Build history of the part. All positions in model axes, mm. A direction names the side the tool comes from. Coordinates: 2 decimals unless noted, no trailing zeros. Write each loop counter-clockwise with the first axis right and the second up, starting at its lowest first coordinate (ties: lowest second). Pieces come first, ordered by that corner, then holes. Notation, with made-up numbers: (18.25, 78) -> (72.25, 78) arc R11 cw to (72.25, 98) -> close; hole circle Ø5 at (0, 82). An arc over 180 degrees is marked (long way). Write each question's results on one line, items separated by ' | '. Start each with the question number.
Q1. Drill centre lines: line 1 (Z direction, x = -4.75, y = 4.75); line 2 (Y direction, x = 2, z = 0); line 3 (Y direction, x = 0.75, z = 0). Where is each one in solid material? Low to high.
Q2. Saw through at A-A on x = 5.5. Give the cut face in (y, z), and give its area (3 significant figures).
Q3. Tool access for faces 1 (the face through (-3.9, 4.7, 1)), 2 (the face through (4, 3, -2.25)), 3 (the face through (0, 0, 0)): list every direction of +Z, -Z, +X, -X, +Y, -Y with a clear straight run to the whole face (end or side of a thin tool).
Q4. Saw through at C-C on x = -3.25. Give the cut face in (y, z).
Q5. Saw through at B-B on y = -0.25. Give the cut face in (x, z).
Q6. Drop a flat-ended pin along its axis: pin 1 Ø1.2 at (x, y) = (-2.5, 2.5) entering from -Z. Give the stop position or say it passes through.
Q7. Two-plate mould, pull along Z, no slides. Class faces 4 (the face through (-4.85, 0.6, 2.5)), 5 (the face through (7.2, 1, -1.5)), 6 (the face through (5, 3, -3.25)), 7 (the face through (-4, 3.8, 2.5)): released by +Z, released by -Z, zero draft, split by the parting line, or undercut.
from build123d import *
from build123d.topology import SkipClean

# Parameters (mm, degrees)
SKETCH1_W                            = 11.7
SKETCH1_H                            = 6.5
BOSS_EXTRUDE1_DEPTH                  = 5.5
SKETCH2_R                            = 1.75
CUT_EXTRUDE1_DEPTH                   = 15.5
BOSS_EXTRUDE2_START                  = 2.6
SKETCH3_R                            = 2.5
SKETCH3_R_2                          = 1.75
BOSS_EXTRUDE2_DEPTH                  = 2.6
CUT_EXTRUDE2_START                   = -1
CUT_EXTRUDE2_DEPTH                   = 9.7
CUT_EXTRUDE3_DEPTH                   = 10
SKETCH6_W                            = 2.5
SKETCH6_H                            = 2
SKETCH6_W_2                          = 2
CUT_EXTRUDE4_DEPTH                   = 2
SKETCH7_W                            = 9.85
SKETCH7_H                            = 4.5
CUT_EXTRUDE5_DEPTH                   = 0.5
FILLET1_R                            = 0.2
SKETCH8_R                            = 0.5
BOSS_EXTRUDE3_DEPTH                  = 1
BOSS_EXTRUDE3_DIRECTION_2_REACH      = 12.593
BOSS_EXTRUDE3_DIRECTION_2_END_RADIUS = 3
FILLET2_R                            = 0.3


with BuildPart() as part:
    # Sketch1 → Boss-Extrude1 (new body)
    with BuildSketch(Plane(origin=(0, 0, 0), x_dir=(1, 0, 0), z_dir=(0, 1, 0))):
        Rectangle(SKETCH1_W, SKETCH1_H)
    extrude(amount=BOSS_EXTRUDE1_DEPTH)

    # Sketch2 → Cut-Extrude1 (cut)
    with BuildSketch(Plane(origin=(5.85, 0, 0), x_dir=(0, 0, -1), z_dir=(1, 0, 0))):
        with Locations((0, 3)):
            Circle(SKETCH2_R)
    extrude(amount=-CUT_EXTRUDE1_DEPTH, mode=Mode.SUBTRACT)

    # Sketch3 → Boss-Extrude2 (add)
    with BuildSketch(Plane(origin=(5.85, 0, 0), x_dir=(0, 0, -1), z_dir=(1, 0, 0)).offset(BOSS_EXTRUDE2_START)):
        with Locations(Location((0, 3, 0), (0, 0, 90))):
            Circle(SKETCH3_R)
        with Locations((0, 3)):
            Circle(SKETCH3_R_2, mode=Mode.SUBTRACT)
    extrude(amount=-BOSS_EXTRUDE2_DEPTH)

    # Sketch4 → Cut-Extrude2 (cut)
    with BuildSketch(Plane(origin=(5.85, 0, 0), x_dir=(0, 0, -1), z_dir=(1, 0, 0)).offset(CUT_EXTRUDE2_START)):
        with BuildLine():
            Line((-4.687033743, 2), (-2.828427125, 2))
            ThreePointArc((-2.828427125, 2), (0, 0), (2.828427125, 2))
            Line((2.828427125, 2), (5.329187563, 2))
            Line((5.329187563, 2), (5.329187563, -1.490759496))
            Line((5.329187563, -1.490759496), (-4.687033743, -1.490759496))
            Line((-4.687033743, -1.490759496), (-4.687033743, 2))
        make_face()
    extrude(amount=-CUT_EXTRUDE2_DEPTH, mode=Mode.SUBTRACT)

    # Sketch5 → Cut-Extrude3 (cut)
    with BuildSketch(Plane(origin=(0, 5.5, 0), x_dir=(1, 0, 0), z_dir=(0, 1, 0))):
        Polygon((-3.5, 4.45), (-2, 4.45), (-2, 2.75), (-1.5, 2.75), (-1.5, 2.25), (-4, 2.25), (-4, 2.75), (-3.5, 2.75), align=None)
        Polygon((0.3, 4.45), (1.3, 4.45), (1.3, 2.75), (1.8, 2.75), (1.8, 2.25), (-0.2, 2.25), (-0.2, 2.75), (0.3, 2.75), align=None)
        Polygon((3.6, 4.45), (4.6, 4.45), (4.6, 2.75), (5.1, 2.75), (5.1, 2.25), (3.1, 2.25), (3.1, 2.75), (3.6, 2.75), align=None)
        Polygon((1.3, -2.75), (1.8, -2.75), (1.8, -2.25), (-0.2, -2.25), (-0.2, -2.75), (0.3, -2.75), (0.3, -4.45), (1.3, -4.45), align=None)
        Polygon((-2, -2.75), (-1.5, -2.75), (-1.5, -2.25), (-4, -2.25), (-4, -2.75), (-3.5, -2.75), (-3.5, -4.45), (-2, -4.45), align=None)
        Polygon((5.1, -2.25), (5.1, -2.75), (4.6, -2.75), (4.6, -4.45), (3.6, -4.45), (3.6, -2.75), (3.1, -2.75), (3.1, -2.25), align=None)
    extrude(amount=-CUT_EXTRUDE3_DEPTH, mode=Mode.SUBTRACT)

    # Sketch6 → Cut-Extrude4 (cut)
    with BuildSketch(Plane(origin=(0, 5.5, 0), x_dir=(1, 0, 0), z_dir=(0, 1, 0))):
        with Locations((-3.63, 0)):
            Rectangle(SKETCH6_W, SKETCH6_H)
        with Locations((0.9, 0)):
            Rectangle(SKETCH6_W_2, SKETCH6_H)
        with Locations((4.02, 0)):
            Rectangle(SKETCH6_W_2, SKETCH6_H)
    extrude(amount=-CUT_EXTRUDE4_DEPTH, mode=Mode.SUBTRACT)

    # Sketch7 → Cut-Extrude5 (cut)
    with BuildSketch(Plane(origin=(0, 5.5, 0), x_dir=(1, 0, 0), z_dir=(0, 1, 0))):
        with Locations((0.925, 0)):
            Rectangle(SKETCH7_W, SKETCH7_H)
    extrude(amount=-CUT_EXTRUDE5_DEPTH, mode=Mode.SUBTRACT)

    # Fillet1
    fillet1_edges = [part.edges().sort_by_distance(p)[0] for p in [
        (-2.75, 5, -2.25),
        (0.8, 5, -2.25),
        (4.1, 5, 2.25),
        (0.8, 5, 2.25),
        (-2.75, 5, 2.25),
        (4.1, 5, -2.25),
    ]]
    fillet(fillet1_edges, radius=FILLET1_R)

    # Sketch8 → Boss-Extrude3 (add)
    with BuildSketch(Plane.XZ):
        with Locations(Location((4.05, 0, 0), (0, 0, 90))):
            Circle(SKETCH8_R)
        with Locations(Location((-2.15, 0, 0), (0, 0, 90))):
            Circle(SKETCH8_R)
    extrude(amount=BOSS_EXTRUDE3_DEPTH)

    # Boss-Extrude3 direction 2: up to this cylinder (the profile starts outside it)
    with SkipClean():  # the faces are left unmerged after this step: merging them gives an invalid solid
        boss_extrude3_direction_2_end = Plane(origin=(0.95, 3, 0), z_dir=(1, 0, 0)) * Cylinder(BOSS_EXTRUDE3_DIRECTION_2_END_RADIUS, 38.386, mode=Mode.PRIVATE)
        # Sketch8 → Boss-Extrude3 direction 2 (add, up to the surface)
        with BuildSketch(Plane.XZ, mode=Mode.PRIVATE) as boss_extrude3_direction_2_sk1:
            with Locations(Location((4.05, 0, 0), (0, 0, 90))):
                Circle(SKETCH8_R)
        boss_extrude3_direction_2_tool1 = extrude(boss_extrude3_direction_2_sk1.sketch, amount=-BOSS_EXTRUDE3_DIRECTION_2_REACH, mode=Mode.PRIVATE) - boss_extrude3_direction_2_end
        add(boss_extrude3_direction_2_tool1.solids().sort_by_distance((4.05, 0, 0))[0])
        add(boss_extrude3_direction_2_tool1.solids().sort_by_distance((4.05, 0, 0))[1])
        # Sketch8 → Boss-Extrude3 direction 2 (add, up to the surface)
        with BuildSketch(Plane.XZ, mode=Mode.PRIVATE) as boss_extrude3_direction_2_sk2:
            with Locations(Location((-2.15, 0, 0), (0, 0, 90))):
                Circle(SKETCH8_R)
        boss_extrude3_direction_2_tool2 = extrude(boss_extrude3_direction_2_sk2.sketch, amount=-BOSS_EXTRUDE3_DIRECTION_2_REACH, mode=Mode.PRIVATE) - boss_extrude3_direction_2_end
        add(boss_extrude3_direction_2_tool2.solids().sort_by_distance((-2.15, 0, 0))[0])
        add(boss_extrude3_direction_2_tool2.solids().sort_by_distance((-2.15, 0, 0))[1])

    # Fillet2
    fillet2_edges = [part.edges().sort_by_distance(p)[0] for p in [
        (4.05, -1, -0.5),
        (-2.15, -1, -0.5),
    ]]
    fillet(fillet2_edges, radius=FILLET2_R)


solid = part.part
Returned:
1) line 1: z = -3.25 to -1, 1 to 3.25 | line 2: y = 0 to 1.25, 4.75 to 5 | line 3: y = 0 to 1.25
2) outline: (0, -3.25) -> (5.5, -3.25) -> (5.5, -2.25) -> (5, -2.25) -> (5, 2.25) -> (5.5, 2.25) -> (5.5, 3.25) -> (0, 3.25) -> close; hole circle Ø3.5 at (3, 0) | area: 23.9 mm2
3) face 1: +Y | face 2: +Y, -Y | face 3: -Y
4) outline: (1.02, -2.25) -> (4.8, -2.25) arc R0.2 ccw to (5, -2.05) -> (5, -1) -> (4.44, -1) arc R1.75 cw (long way) to (4.44, 1) -> (5, 1) -> (5, 2.05) arc R0.2 ccw to (4.8, 2.25) -> (1.02, 2.25) arc R3 ccw to start
5) outline: circle Ø1 at (-2.15, 0); circle Ø1 at (4.05, 0)
6) pin 1: stops at z = -3.25
7) face 4: zero draft | face 5: split by the parting line | face 6: released by -Z | face 7: undercut
